The listing builds one solid part. Answer for the finished solid, in the listing's coordinates (mm). A direction names the side the tool comes from. Round coordinates to 2 decimals unless told otherwise and drop trailing zeros. Write each loop counter-clockwise with the first axis right and the second up, starting at its lowest first coordinate (ties: lowest second). Pieces come first, ordered by that corner, then holes. Notation, with made-up numbers: (65.25, 26.25) - (71.25, 26.25) arc R19 ccw to (71.25, 33.25) - close; hole circle Ø6 at (4, 16.25). An arc over 180 degrees is marked (long way). Return JSON: item names as keys, results as strings. Group by question number.
(1) Section D-D, the plane z = 15 is taken. Give the number of separate pieces and of enclosed holes in the cut face, then the cut area to 3 significant figures.
(2) Section A-A, the plane z = 0 is taken. Write down the section's boundary in (x, y), then the cut area to 3 significant figures.
(3) Each of these flat-tipped pins is pushed along its axis until it touches: pin 1 (3 mm diameter, centred on y = 9, z = -5, fed in from +X); pin 2 (10 mm diameter, centred on x = -14.5, y = 17.5, fed in from -Z); pin 3 (1.5 mm diameter, centred on x = -20.5, y = 4, fed in from -Z); pin 4 (12 mm diameter, centred on x = -21, z = 4, fed in from +Y). Where does it stop, or does it pass through?
(4) Determine the mould class of faces 3 (the cylindrical face through (-5.961, 9.633, 26.846)), 4 (the flat face through (20, 20, -16)), 5 (the cylindrical face through (15.75, 6.66, 11.61)) for opening direction X: +X half, -X half, draft (parallel to the pull), parting line (faces both ways), or undercut.
(5) Section C-C, the plane y = 2.5 is taken. Write down the section's boundary in (x, z).
(6) Find the intervals of material crossed by line 1 along X through (y, z) = (15.5, 0); line 2 along X through (y, z) = (9.5, 14); line 3 along X through (y, z) = (1.75, 12), in increasing order. Write a range as [from, to].
(7) Section B-B, the plane x = 0 is taken. Write down the section's boundary in (y, z), then the cut area to 3 significant figures.
(8) Which of the six approach directions +Z, -Z, +X, -X, +Y, -Y give full straight-line access (tool end or side, diameter ignored) to faces 1 (the cylindrical face through (17.004, 6.656, -15.043)), 2 (the cylindrical face through (23.846, 16.704, -7.509))?
```python
from build123d import *

# Parameters (mm, degrees)
SKETCH2_R               = 3
CUT_EXTRUDE2_DEPTH      = 21
CUT_EXTRUDE2_DEPTH_BACK = 1
CHAMFER1_SIZE           = 1


with BuildPart() as part:
    # Sketch1 → Revolve1 (revolve)
    with BuildSketch(Plane.XY):
        Polygon((27.5, 0), (27.5, 20), (25, 20), (25, 13.5), (0, 13.5), (0, 0), align=None)
    revolve(axis=Axis((0, -626.687351978, 0), (0, 1, 0)))

    # Sketch2 → Cut-Extrude2 (cut, two sides)
    with BuildSketch(Plane(origin=(0, 0, 0), x_dir=(1, 0, 0), z_dir=(0, 1, 0))) as cut_extrude2_sk:
        with Locations((-14.142135624, 14.142135624)):
            Circle(SKETCH2_R)
        with Locations((14.142135624, 14.142135624)):
            Circle(SKETCH2_R)
        with Locations((14.142135624, -14.142135624)):
            Circle(SKETCH2_R)
        with Locations((-14.142135624, -14.142135624)):
            Circle(SKETCH2_R)
    extrude(amount=CUT_EXTRUDE2_DEPTH, mode=Mode.SUBTRACT)
    extrude(cut_extrude2_sk.sketch, amount=-CUT_EXTRUDE2_DEPTH_BACK, mode=Mode.SUBTRACT)

    # Chamfer1
    chamfer1_edges = [part.edges().sort_by_distance(p)[0] for p in [
        (-27.5, 20, 0),
    ]]
    chamfer(chamfer1_edges, length=CHAMFER1_SIZE)


solid = part.part
```
Working result:
{
 "1": {"separate pieces": "3", "enclosed holes": "0", "area": "506 mm^2"},
 "2": {"outline": "(-27.5, 0) - (27.5, 0) - (27.5, 19) - (26.5, 20) - (25, 20) - (25, 13.5) - (-25, 13.5) - (-25, 20) - (-26.5, 20) - (-27.5, 19) - close", "area": "774 mm^2"},
 "3": {"pin 1": "stops at x = 27.28", "pin 2": "stops at z = -25.81", "pin 3": "stops at z = -19.14", "pin 4": "stops at y = 20"},
 "4": {"face 3": "parting line", "face 4": "draft", "face 5": "undercut"},
 "5": {"outline": "circle Ø55 at (0, 0); hole circle Ø6 at (-14.14, -14.14); hole circle Ø6 at (-14.14, 14.14); hole circle Ø6 at (14.14, -14.14); hole circle Ø6 at (14.14, 14.14)"},
 "6": {"line 1": "x = [-27.5, -25], [25, 27.5]", "line 2": "x = [-23.67, -17.14], [-11.15, 11.15], [17.14, 23.67]", "line 3": "x = [-24.74, -16.24], [-12.04, 12.04], [16.24, 24.74]"},
 "7": {"outline": "(0, -27.5) - (19, -27.5) - (20, -26.5) - (20, -25) - (13.5, -25) - (13.5, 25) - (20, 25) - (20, 26.5) - (19, 27.5) - (0, 27.5) - close", "area": "774 mm^2"},
 "8": {"face 1": "+Y, -Y", "face 2": "+Y"}
}
